Input: part model. Units: mm. Frame: model coordinates. Face numbers are marked on the shaded views. A direction names the side the tool comes from. Round coordinates to 2 decimals unless told otherwise and drop trailing zeros. Loops run counter-clockwise (first coordinate to the right, second up) from the corner with the lowest first, then second, coordinate; pieces in that order, holes last. Notation, with made-up numbers: (3.25, -23.5) -> (22.25, -23.5) arc R18 ccw to (22.25, -6.5) -> close; hole circle Ø10 at (64.5, 62). An arc over 180 degrees is marked (long way). Answer as a JSON object with one key per item and string values. Group by question number.
Item 1: Set-up query: the marked faces 1 and 2. Return all of +Z, -Z, +X, -X, +Y, -Y with unobstructed straight access to the full face (end or side cutting, diameter ignored); none if empty.
Item 2: Section query C-C on z = 117. Return loops of the section in (x, y), and give its area (3 significant figures).
Item 3: Material intervals for line 1 (Z direction, x = -7.5, y = -51); line 2 (Z direction, x = -14, y = -38.5); line 3 (Z direction, x = -8, y = -88), sorted ascending. Write a range as [from, to].
Item 4: Section query D-D on y = -44.5. Return loops of the section in (x, z), and give its area (3 significant figures).
Item 5: Section query B-B on x = -28.5. Return loops of the section in (y, z), and give its area (3 significant figures).
Item 6: Draft query along Z for the marked faces 3 and 4. Return one class per face: released by +Z, released by -Z, zero draft, split by the parting line, or undercut.
Item 7: Pin query (flat end, axial travel): pin 1 (6 mm diameter, centred on x = 19, y = -81, fed in from -Z); pin 2 (6 mm diameter, centred on x = 3.5, y = -67.5, fed in from +Z); pin 3 (10 mm diameter, centred on x = -20, y = -75, fed in from -Z). Return the tip coordinate at first contact, or that it passes through.
Item 8: Section query A-A on y = -23. Return loops of the section in (x, z).
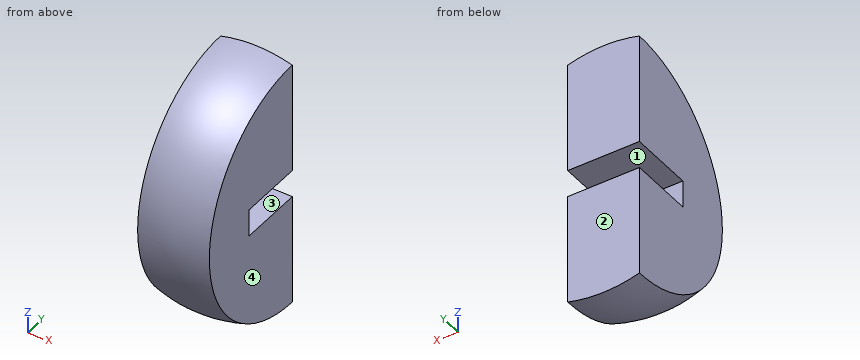
from build123d import *

# Parameters (mm, degrees)
CUT_EXTRUDE2_START       = -135
CUT_EXTRUDE2_OUTLINE_W   = 131
CUT_EXTRUDE2_OUTLINE_H   = 262
CUT_EXTRUDE2_DEPTH       = 97.5
CUT_EXTRUDE2_START_2     = 37.5
CUT_EXTRUDE2_2_OUTLINE_W = 131
CUT_EXTRUDE2_2_OUTLINE_H = 262
CUT_EXTRUDE2_2_DEPTH     = 97.5
SKETCH3_W                = 37.5
SKETCH3_H                = 28.5
CUT_EXTRUDE3_DEPTH       = 68


# Read off the part's stored shape, not the designer's step: Cut-Extrude2
with BuildPart() as part:
    # Sketch1 → Revolve2 (revolve)
    with BuildSketch(Plane.XY, mode=Mode.PRIVATE) as revolve2_sk:
        with BuildLine():
            Line((135, 0), (0, 0))
            Line((0, 0), (0, -135))
            ThreePointArc((0, -135), (95.45941546, -95.45941546), (135, 0))
        make_face()
    revolve(revolve2_sk.sketch.rotate(Axis((0, 0, 0), (0, 1, 0)), 180), axis=Axis((0, 0, 0), (0, 1, 0)))

    # Cut-Extrude2 outline → Cut-Extrude2 (cut)
    with BuildSketch(Plane.YZ.offset(CUT_EXTRUDE2_START)):
        with Locations((-65.5, 0)):
            Rectangle(CUT_EXTRUDE2_OUTLINE_W, CUT_EXTRUDE2_OUTLINE_H)
    extrude(amount=CUT_EXTRUDE2_DEPTH, mode=Mode.SUBTRACT)

    # Cut-Extrude2 2 outline → Cut-Extrude2 2 (cut)
    with BuildSketch(Plane.YZ.offset(CUT_EXTRUDE2_START_2)):
        with Locations((-65.5, 0)):
            Rectangle(CUT_EXTRUDE2_2_OUTLINE_W, CUT_EXTRUDE2_2_OUTLINE_H)
    extrude(amount=CUT_EXTRUDE2_2_DEPTH, mode=Mode.SUBTRACT)

    # Sketch3 → Cut-Extrude3 (cut)
    with BuildSketch(Plane(origin=(0, 0, 0), x_dir=(1, 0, 0), z_dir=(0, 1, 0))):
        with Locations((18.75, 0)):
            Rectangle(SKETCH3_W, SKETCH3_H)
        with Locations((-18.75, 0)):
            Rectangle(SKETCH3_W, SKETCH3_H)
    extrude(amount=-CUT_EXTRUDE3_DEPTH, mode=Mode.SUBTRACT)


solid = part.part
Solved:
{
 "1": {"face 1": "+X, -X, +Y", "face 2": "+Z, -Z, +X, -X, +Y"},
 "2": {"outline": "(-37.5, -55.94) arc R67.35 ccw to (37.5, -55.94) -> (37.5, 0) -> (-37.5, 0) -> close", "area": "4,780 mm²"},
 "3": {"line 1": "[-124.77, -14.25], [14.25, 124.77]", "line 2": "[-128.63, -14.25], [14.25, 128.63]", "line 3": "[-102.06, 102.06]"},
 "4": {"outline": "(-37.5, -121.81) arc R127.45 ccw to (37.5, -121.81) -> (37.5, -14.25) -> (-37.5, -14.25) -> close; (-37.5, 14.25) -> (37.5, 14.25) -> (37.5, 121.81) arc R127.45 ccw to (-37.5, 121.81) -> close", "area": "16,700 mm²"},
 "5": {"outline": "(-68, -14.25) -> (-68, 14.25) -> (0, 14.25) -> (0, 131.96) arc R131.96 ccw to (0, -131.96) -> (0, -14.25) -> close", "area": "25,400 mm²"},
 "6": {"face 3": "undercut", "face 4": "zero draft"},
 "7": {"pin 1": "z = -108.6", "pin 2": "z = 118.55", "pin 3": "z = -113.8"},
 "8": {"outline": "(-37.5, -127.63) arc R133.03 ccw to (37.5, -127.63) -> (37.5, -14.25) -> (-37.5, -14.25) -> close; (-37.5, 14.25) -> (37.5, 14.25) -> (37.5, 127.63) arc R133.03 ccw to (-37.5, 127.63) -> close"}
}
